Part model, mm, in its own coordinate system. A direction names the side the tool comes from. Round coordinates to 2 decimals unless told otherwise and drop trailing zeros. Loops run counter-clockwise (first coordinate to the right, second up) from the corner with the lowest first, then second, coordinate; pieces in that order, holes last.
(1) Tool access for faces 5 (the face through (-8, 12, 2)), 6 (the face through (34, 9.5, 6.9)), 7 (the face through (31.5, -15, 28)), 8 (the face through (12, -12, 2)): list every direction of +Z, -Z, +X, -X, +Y, -Y with a clear straight run to the whole face (end or side of a thin tool).
(2) Cut at C-C on x = 17.5. List the corners of the cut face in (y, z), then the cut area to 3 significant figures.
(3) Cut at B-B on z = 35.1. List the corners of the cut face in (x, y), then the cut area to 3 significant figures.
(4) Flat gauge pins, fed straight in: pin 1 (10 mm diameter, centred on x = 9, z = 7.5, fed in from -Y); pin 2 (2.5 mm diameter, centred on y = -14.5, z = 35.1, fed in from -X); pin 3 (3.5 mm diameter, centred on x = -12.5, z = 1.5, fed in from +Y); pin 4 (5 mm diameter, centred on y = -14.5, z = 20.1, fed in from -X). Where does each tip first touch, or does it go through?
(5) Cut at A-A on y = -5.5. List the corners of the cut face in (x, z).
(6) Cut at D-D on y = 9. List the corners of the cut face in (x, z), then the cut area to 3 significant figures.
(7) Probe probe 1 along Y at (x, z) = (37, 15.1); probe 2 along Z at (x, y) = (34.75, 14.5); probe 3 along X at (y, z) = (-4.5, 3). List the from-to ranges inside material, lowest first.
(8) Mould opens along Z. For faces 1 (the face through (35.44, 14.05, 23.67)), 2 (the face through (35.44, -14.95, 23.67)), 3 (the face through (-26, -12, 2)), 4 (the face through (36, -15, 38.6)) say: +Z half, -Z half, draft (parallel to the pull), parting line (faces both ways), or undercut.
Autodesk Inventor part; units mm, degrees
ref_plane "YZ Plane" through (0, 0, 0) normal (1, 0, 0) x (0, 1, 0)
ref_plane "XZ Plane" through (0, 0, 0) normal (0, 1, 0) x (-1, 0, 0)
ref_plane "XY Plane" through (0, 0, 0) normal (0, 0, 1) x (1, 0, 0)
sketch "Sketch1" plane through (0, 0, 0) normal (0, 0, 1) x (1, 0, 0)
  line L0 (-39.5, 12) -> (39.5, 12)
  line L1 (39.5, 12) -> (39.5, -12)
  line L2 (39.5, -12) -> (-39.5, -12)
  line L3 (-39.5, -12) -> (-39.5, 12)
  line L4 (-39.5, 12) -> (39.5, -12) construction
  line L5 (39.5, 12) -> (-39.5, -12) construction
  point P0 (0, 0)
  dimension "d0" = 79
  dimension "d1" = 24
extrude "Extrusion1" add sketch "Sketch1" along normal blind 4.4
sketch "Sketch3" plane through (0, 0, 0) normal (0, 0, -1) x (-1, 0, 0)
  line L0 (-39.5, 12) -> (-31.5, 12)
  line L1 (-31.5, 12) -> (-31.5, 18.5)
  line L2 (-31.5, 18.5) -> (-39.5, 18.5)
  line L3 (-39.5, 18.5) -> (-39.5, 12)
  line L4 (-39.5, -12) -> (-31.5, -12)
  line L5 (-31.5, -12) -> (-31.5, -18.5)
  line L6 (-31.5, -18.5) -> (-39.5, -18.5)
  line L7 (-39.5, -18.5) -> (-39.5, -12)
  point P0 (0, 0)
  dimension "d8" = 8
  dimension "d9" = 6.5
  dimension "d10" = 6.5
extrude "Extrusion2" add sketch "Sketch3" against normal blind 38.6
chamfer "Chamfer1" distance 6.5 angle 45 2 edges at (31.5, -12, 2.2) (31.5, 12, 2.2)
sketch "Sketch5" plane through (0, 0, 0) normal (0, 0, -1) x (-1, 0, 0)
  line L0 (-25, -12) -> (39.5, -12)
  line L1 (39.5, 12) -> (-24.5, 12) construction
  line L2 (-24.5, 12) -> (-24.5, -12) construction
  line L3 (-24.5, -12) -> (39.5, -12) construction
  line L4 (39.5, -12) -> (39.5, 12) construction
  line L5 (-24.5, 12) -> (39.5, -12) construction
  line L6 (39.5, 12) -> (-24.5, -12) construction
  circle A0 centre (7.5, 0) radius 6.1
  line L7 (-17.5, 3) -> (32.5, 3) construction
  line L8 (32.5, 3) -> (32.5, -3) construction
  line L9 (32.5, -3) -> (-17.5, -3) construction
  line L10 (-17.5, -3) -> (-17.5, 3) construction
  line L11 (-17.5, 3) -> (32.5, -3) construction
  line L12 (32.5, 3) -> (-17.5, -3) construction
  circle A1 centre (-17.5, 0) radius 2.4
  circle A2 centre (32.5, 0) radius 2.4
  line L13 (1.4, 0) -> (1.4, -12)
  line L14 (13.6, 0) -> (13.6, -12)
  line L15 (13.6, -12) -> (1.4, -12)
  point P0 (0, 0)
  dimension "d29" = 64
  dimension "d30" = 12.2
  dimension "d31" = 50
  dimension "d32" = 4.8
  dimension "d33" = 4.8
extrude "Extrusion4" cut sketch "Sketch5" against normal blind 5.6
sketch "Sketch6" plane through (39.5, -18.5, 0) normal (1, 0, 0) x (0, 0, -1)
  line L0 (-38.6, 6.5) -> (-5.6, 6.5) construction
  line L1 (-5.6, 6.5) -> (-5.6, 1.5) construction
  line L2 (-5.6, 1.5) -> (-38.6, 1.5) construction
  line L3 (-38.6, 1.5) -> (-38.6, 6.5) construction
  line L4 (-38.6, 30.5) -> (-5.6, 30.5) construction
  line L5 (-5.6, 30.5) -> (-5.6, 35.5) construction
  line L6 (-5.6, 35.5) -> (-38.6, 35.5) construction
  line L7 (-38.6, 35.5) -> (-38.6, 30.5) construction
  line L8 (-38.6, 4) -> (-5.6, 4) construction
  line L9 (-38.6, 33) -> (-5.6, 33) construction
  line L10 (-38.6, 1.5) -> (-37.6, 1.5) construction
  line L11 (-37.6, 1.5) -> (-37.6, 6.5) construction
  line L12 (-37.6, 6.5) -> (-38.6, 6.5) construction
  line L13 (-38.6, 6.5) -> (-38.6, 1.5) construction
  line L14 (-37.6, 1.5) -> (-32.6, 1.5) construction
  line L15 (-32.6, 1.5) -> (-32.6, 6.5) construction
  line L16 (-32.6, 6.5) -> (-37.6, 6.5) construction
  line L17 (-37.6, 6.5) -> (-37.6, 1.5) construction
  line L18 (-38.6, 30.5) -> (-37.6, 30.5) construction
  line L19 (-37.6, 30.5) -> (-37.6, 35.5) construction
  line L20 (-37.6, 35.5) -> (-38.6, 35.5) construction
  line L21 (-38.6, 35.5) -> (-38.6, 30.5) construction
  line L22 (-37.6, 30.5) -> (-32.6, 30.5) construction
  line L23 (-32.6, 30.5) -> (-32.6, 35.5) construction
  line L24 (-32.6, 35.5) -> (-37.6, 35.5) construction
  line L25 (-37.6, 35.5) -> (-37.6, 30.5) construction
  line L26 (-37.6, 1.5) -> (-32.6, 6.5) construction
  line L27 (-37.6, 6.5) -> (-32.6, 1.5) construction
  line L28 (-37.6, 30.5) -> (-32.6, 35.5) construction
  line L29 (-37.6, 35.5) -> (-32.6, 30.5) construction
  line L30 (-38.6, 35.5) -> (-37.6, 35.5) construction
  line L31 (-37.6, 35.5) -> (-37.6, 30.5) construction
  line L32 (-37.6, 30.5) -> (-38.6, 30.5) construction
  line L33 (-38.6, 30.5) -> (-38.6, 35.5) construction
  line L34 (-4.4, 30.5) -> (-38.6, 30.5)
  line L35 (-32.6, 35.5) -> (-27.6, 35.5) construction
  line L36 (-27.6, 35.5) -> (-27.6, 30.5) construction
  line L37 (-27.6, 30.5) -> (-32.6, 30.5) construction
  line L38 (-32.6, 30.5) -> (-32.6, 35.5) construction
  line L39 (-27.6, 35.5) -> (-22.6, 35.5) construction
  line L40 (-22.6, 35.5) -> (-22.6, 30.5) construction
  line L41 (-22.6, 30.5) -> (-27.6, 30.5) construction
  line L42 (-27.6, 30.5) -> (-27.6, 35.5) construction
  line L43 (-32.6, 6.5) -> (-27.6, 6.5) construction
  line L44 (-27.6, 6.5) -> (-27.6, 1.5) construction
  line L45 (-27.6, 1.5) -> (-32.6, 1.5) construction
  line L46 (-32.6, 1.5) -> (-32.6, 6.5) construction
  line L47 (-27.6, 6.5) -> (-22.6, 6.5) construction
  line L48 (-22.6, 6.5) -> (-22.6, 1.5) construction
  line L49 (-22.6, 1.5) -> (-27.6, 1.5) construction
  line L50 (-27.6, 1.5) -> (-27.6, 6.5) construction
  line L51 (-22.6, 35.5) -> (-17.6, 35.5) construction
  line L52 (-17.6, 35.5) -> (-17.6, 30.5) construction
  line L53 (-17.6, 30.5) -> (-22.6, 30.5) construction
  line L54 (-22.6, 30.5) -> (-22.6, 35.5) construction
  line L55 (-22.6, 6.5) -> (-17.6, 6.5) construction
  line L56 (-17.6, 6.5) -> (-17.6, 1.5) construction
  line L57 (-17.6, 1.5) -> (-22.6, 1.5) construction
  line L58 (-22.6, 1.5) -> (-22.6, 6.5) construction
  line L59 (-17.6, 35.5) -> (-12.6, 35.5) construction
  line L60 (-12.6, 35.5) -> (-12.6, 30.5) construction
  line L61 (-12.6, 30.5) -> (-17.6, 30.5) construction
  line L62 (-17.6, 30.5) -> (-17.6, 35.5) construction
  line L63 (-17.6, 6.5) -> (-12.6, 6.5) construction
  line L64 (-12.6, 6.5) -> (-12.6, 1.5) construction
  line L65 (-12.6, 1.5) -> (-17.6, 1.5) construction
  line L66 (-17.6, 1.5) -> (-17.6, 6.5) construction
  line L67 (-32.6, 35.5) -> (-27.6, 30.5) construction
  line L68 (-27.6, 35.5) -> (-32.6, 30.5) construction
  line L69 (-27.6, 35.5) -> (-22.6, 30.5) construction
  line L70 (-27.6, 30.5) -> (-22.6, 35.5) construction
  line L71 (-22.6, 30.5) -> (-17.6, 35.5) construction
  line L72 (-22.6, 35.5) -> (-17.6, 30.5) construction
  line L73 (-17.6, 35.5) -> (-12.6, 30.5) construction
  line L74 (-12.6, 35.5) -> (-17.6, 30.5) construction
  line L75 (-17.6, 6.5) -> (-12.6, 1.5) construction
  line L76 (-12.6, 6.5) -> (-17.6, 1.5) construction
  line L77 (-22.6, 6.5) -> (-17.6, 1.5) construction
  line L78 (-17.6, 6.5) -> (-22.6, 1.5) construction
  line L79 (-27.6, 6.5) -> (-22.6, 1.5) construction
  line L80 (-22.6, 6.5) -> (-27.6, 1.5) construction
  line L81 (-32.6, 6.5) -> (-27.6, 1.5) construction
  line L82 (-27.6, 6.5) -> (-32.6, 1.5) construction
  point P0 (0, 18.5)
  point P1 (-35.1, 4)
  point P2 (-35.1, 33)
  point P3 (-30.1, 33)
  point P4 (-25.1, 33)
  point P5 (-20.1, 33)
  point P6 (-15.1, 33)
  point P7 (-15.1, 4)
  point P8 (-20.1, 4)
  point P9 (-25.1, 4)
  point P10 (-30.1, 4)
  dimension "d42" = 5
  dimension "d43" = 5
  dimension "d44" = 1
  dimension "d45" = 5
  dimension "d46" = 5
  dimension "d54" = 33
  dimension "d55" = 1
  dimension "d59" = 5
  dimension "d60" = 5
  dimension "d61" = 5
  dimension "d62" = 5
hole "Hole2" at (39.5, -14.5, 35.1) at (39.5, 14.5, 35.1) at (39.5, 14.5, 30.1) at (39.5, 14.5, 25.1) at (39.5, 14.5, 20.1) at (39.5, 14.5, 15.1) at (39.5, -14.5, 15.1) at (39.5, -14.5, 20.1) at (39.5, -14.5, 25.1) at (39.5, -14.5, 30.1) direction (-1, 0, 0) diameter 3 end through all
chamfer "Chamfer2" distance 6.4 angle 45 2 edges at (31.5, 15.25, 4.4) (31.5, -15.25, 4.4)
chamfer "Chamfer3" distance 5 angle 45 2 edges at (35.5, 12, 4.4) (35.5, -12, 4.4)
properties part number "Servo-Groove-Mount-J-Head"
Final values:
1. face 5: +Z, -Z, -X, +Y
1. face 6: +Z, +X, -X
1. face 7: +Z, -X, +Y, -Y
1. face 8: +Z, -Z, -X, -Y
2. outline: (-12, 0) - (-2.4, 0) - (-2.4, 4.4) - (-12, 4.4) - close; (2.4, 0) - (12, 0) - (12, 4.4) - (2.4, 4.4) - close
2. area: 84.5 mm2
3. outline: (31.5, -18.5) - (39.5, -18.5) - (39.5, -16) - (31.5, -16) - close; (31.5, -13) - (39.5, -13) - (39.5, -12) - (31.5, -12) - close; (31.5, 12) - (39.5, 12) - (39.5, 13) - (31.5, 13) - close; (31.5, 16) - (39.5, 16) - (39.5, 18.5) - (31.5, 18.5) - close
3. area: 56.0 mm2
4. pin 1: stops at y = -12
4. pin 2: passes through
4. pin 3: stops at y = 12
4. pin 4: stops at x = 31.5
5. outline: (-39.5, 0) - (-13.6, 0) - (-13.6, 4.4) - (-39.5, 4.4) - close; (-1.4, 0) - (39.5, 0) - (39.5, 4.4) - (-1.4, 4.4) - close
6. outline: (-39.5, 0) - (39.5, 0) - (39.5, 6.4) - (27.1, 6.4) - (25.1, 4.4) - (-39.5, 4.4) - close
6. area: 374 mm2
7. probe 1: y = -18.5 to -16, -13 to -12, 12 to 13, 16 to 18.5
7. probe 2: z = 0 to 13.6, 16.6 to 18.6, 21.6 to 23.6, 26.6 to 28.6, 31.6 to 33.6, 36.6 to 38.6
7. probe 3: x = -39.5 to -13.6, -1.4 to 39.5
8. face 1: undercut
8. face 2: undercut
8. face 3: draft
8. face 4: +Z half
